Geometry: final body of the model. Coordinates: model frame, mm. A direction names the side the tool comes from. Round coordinates to 2 decimals unless told otherwise and drop trailing zeros. Write each loop counter-clockwise with the first axis right and the second up, starting at its lowest first coordinate (ties: lowest second). Pieces come first, ordered by that corner, then holes. Notation, with made-up numbers: M -12.75,9.25 L 20.25,9.25 A20 cw 20.25,35.25 Z; hole C -18.75,10.5 d7. An arc over 180 degrees is marked long. Use one line per item in the form item = value. Start each with the question number.
Item 1: Pin query (flat end, axial travel): pin 1 Ø7.5 at (x, y) = (20.5, 84.5) entering from -Z; pin 2 Ø8.5 at (y, z) = (-40, -71.5) entering from -X; pin 3 Ø6 at (x, z) = (837, 31) entering from +Y; pin 4 Ø4 at (x, y) = (814.5, 1) entering from -Z. Return the tip coordinate at first contact, or that it passes through.
Item 2: Reachability of faces 1 (the flat face through (975, -80, -2)), 2 (the cylindrical face through (493, 31.456, 24.709)) from +Z, -Z, +X, -X, +Y, -Y: full face, straight path, thin tool, end or side. Return the list, or none.
Item 3: Ray query, probe 1 along X at (y, z) = (48, -46.5); probe 2 along Y at (x, z) = (819, -0.5); probe 3 along Y at (x, z) = (594, -32). Return the intervals inside material, ascending.
Item 4: Section query A-A (y = 0). Return loops of the section in (x, z), and give its area (3 significant figures).
Item 5: Pull-direction query (Y, two-part tool) for faces 3 (the flat face through (1000, -46, 2)), 4 (the cylindrical face through (992.605, -23.412, -105.432)), 5 (the flat face through (975, 38, 71)); classes: pulls with the +Y half, pulls with the -Y half, needs draft (parallel to the pull), parting line crosses it, or undercut.
Item 6: Section query B-B (x = 918.5). Return loops of the section in (y, z), and give its area (3 significant figures).
Autodesk Inventor part; units mm, degrees
ref_plane "YZ Plane" through (0, 0, 0) normal (1, 0, 0) x (0, 1, 0)
ref_plane "XZ Plane" through (0, 0, 0) normal (0, 1, 0) x (-1, 0, 0)
ref_plane "XY Plane" through (0, 0, 0) normal (0, 0, 1) x (1, 0, 0)
sketch "Skizze1" plane through (0, 0, 0) normal (1, 0, 0) x (0, 1, 0)
  circle A0 centre (0, 0) radius 40
  circle A1 centre (0, 0) radius 108
  dimension "d0" = 216
  dimension "d1" = 80
extrude "Extrusion1" add sketch "Skizze1" along normal blind 15
sketch "Skizze2" plane through (15, 0, 0) normal (1, 0, 0) x (0, 0, -1)
  circle A0 centre (0, 0) radius 40
  circle A1 centre (0, 0) radius 50
  dimension "d4" = 100
extrude "Extrusion2" add sketch "Skizze2" along normal blind 485
fillet "Rundung1" radius 10 1 edges at (15, 0, 50)
sketch "Skizze3" plane through (15, 0, 0) normal (1, 0, 0) x (0, 0, -1)
  circle A0 centre (0, -85) radius 10 construction
  line L0 (0, -95) -> (-8.7647, -89.8146)
  line L1 (-8.7647, -80.1854) -> (0, -75)
  line L2 (0, -75) -> (8.7647, -80.1854)
  line L3 (8.7647, -80.1854) -> (8.7647, -89.8146)
  line L4 (0, -95) -> (8.7647, -89.8146)
  line L5 (-8.7647, -80.1854) -> (-8.7647, -89.8146)
  point P0 (0, 0)
  dimension "d8" = 20
  dimension "d9" = 85
extrude "Extrusion3" add sketch "Skizze3" along normal blind 10
sketch "Skizze4" plane through (25, 0, 0) normal (1, 0, 0) x (0, 0, -1)
  circle A0 centre (0, -85) radius 5
  point P0 (0, 0)
  dimension "d12" = 10
extrude "Extrusion4" add sketch "Skizze4" along normal blind 10
pattern_circular "Runde Anordnung1" count 6 over 360 about axis through (-10, 0, 0) along (1, 0, 0) of "Extrusion3", "Extrusion4"
mirror "Spiegeln1" about plane through (500, 0, 0) normal (1, 0, 0) of "Extrusion3", "Extrusion4", "Runde Anordnung1", "Extrusion2", "Extrusion1", "Rundung1"
properties part number "DN80-1m"
Working result:
q1.pin_1 = -8.76
q1.pin_2 = 0
q1.pin_3 = 41.42
q1.pin_4 = -50
q2.face_1 = none
q2.face_2 = +X, -X
q3.probe_1 = 0 to 15, 985 to 1000
q3.probe_2 = -50 to -40, 40 to 50
q3.probe_3 = -38.42 to -24, 24 to 38.42
q4.outline = M 0,-108 L 15,-108 L 15,-60 A10 cw 25,-50 L 975,-50 A10 cw 985,-60 L 985,-108 L 1000,-108 L 1000,-40 L 0,-40 Z; M 0,40 L 1000,40 L 1000,108 L 985,108 L 985,60 A10 cw 975,50 L 25,50 A10 cw 15,60 L 15,108 L 0,108 Z
q4.area = 23,600 mm²
q5.face_3 = needs draft
q5.face_4 = parting line crosses it
q5.face_5 = undercut
q6.outline = C 0,0 d100; hole C 0,0 d80
q6.area = 2,830 mm²
